Here's how the part is built. I have some questions about the finished solid (model axes, mm). Round coordinates to 2 decimals unless told otherwise and drop trailing zeros. Loops run counter-clockwise (first coordinate to the right, second up) from the corner with the lowest first, then second, coordinate; pieces in that order, holes last. Notation, with made-up numbers: M 70.25,-17.75 L 117.25,-17.75 A19 cw 117.25,5.25 Z; hole C 30,76.25 d4. An arc over 180 degrees is marked long. Use a Markdown table: item, result.
from build123d import *

# Parameters (mm, degrees)
F0_R     = 57.15
F0_R_2   = 20.32
F0_R_3   = 2.54
F1_DEPTH = 3.175


with BuildPart() as f1:
    # F0 (on Front) → F1 (new body)
    with BuildSketch(Plane.XZ):
        Circle(F0_R)
        with BuildLine():
            Line((-42.883825, -24.53093), (-42.543459, -17.032195))
            ThreePointArc((-42.543459, -17.032195), (-39.820724, -19.644048), (-36.333463, -21.084213))
            Line((-36.333463, -21.084213), (-42.883825, -24.53093))
        make_face(mode=Mode.SUBTRACT)
        with BuildLine():
            Line((-52.656993, -14.806859), (-48.735586, -8.406121))
            ThreePointArc((-48.735586, -8.406121), (-47.587931, -11.928695), (-45.255162, -14.806859))
            Line((-45.255162, -14.806859), (-52.656993, -14.806859))
        make_face(mode=Mode.SUBTRACT)
        with BuildLine():
            Line((-28.536372, -27.7573), (-32.257507, -21.238095))
            ThreePointArc((-32.257507, -21.238095), (-28.390723, -22.188544), (-24.455277, -21.582207))
            Line((-24.455277, -21.582207), (-28.536372, -27.7573))
        make_face(mode=Mode.SUBTRACT)
        with BuildLine():
            Line((-11.408226, -22.576399), (-18.505276, -20.131249))
            ThreePointArc((-18.505276, -20.131249), (-14.403329, -18.445306), (-11.408226, -15.174568))
            Line((-11.408226, -15.174568), (-11.408226, -22.576399))
        make_face(mode=Mode.SUBTRACT)
        with BuildLine():
            Line((-2.212769, -11.019517), (-9.630398, -12.170889))
            ThreePointArc((-9.630398, -12.170889), (-7.613739, -8.986542), (-6.894672, -5.286552))
            Line((-6.894672, -5.286552), (-2.212769, -11.019517))
        make_face(mode=Mode.SUBTRACT)
        with BuildLine():
            Line((-55.724405, 0), (-49.719241, 4.503874))
            ThreePointArc((-49.719241, 4.503874), (-50.727289, 0.088311), (-49.719241, -4.327252))
            Line((-49.719241, -4.327252), (-55.724405, 0))
        make_face(mode=Mode.SUBTRACT)
        with BuildLine():
            Line((-51.745173, 14.383817), (-44.247499, 14.746812))
            ThreePointArc((-44.247499, 14.746812), (-47.252569, 11.671197), (-48.718844, 7.628934))
            Line((-48.718844, 7.628934), (-51.745173, 14.383817))
        make_face(mode=Mode.SUBTRACT)
        with BuildLine():
            Line((-42.743142, 24.165609), (-36.361622, 20.213004))
            ThreePointArc((-36.361622, 20.213004), (-39.870209, 19.076412), (-42.743142, 16.763777))
            Line((-42.743142, 16.763777), (-42.743142, 24.165609))
        make_face(mode=Mode.SUBTRACT)
        with Locations((-28.347915, 0)):
            Circle(F0_R_2, mode=Mode.SUBTRACT)
        with BuildLine():
            Line((-2.37326, 7.45949), (-6.511062, 1.196466))
            ThreePointArc((-6.511062, 1.196466), (-6.73835, 6.076043), (-9.213608, 10.287341))
            Line((-9.213608, 10.287341), (-2.37326, 7.45949))
        make_face(mode=Mode.SUBTRACT)
        with BuildLine():
            Line((-12.167714, 22.883349), (-12.55219, 15.386746))
            ThreePointArc((-12.55219, 15.386746), (-15.311854, 18.527025), (-19.101316, 20.292545))
            Line((-19.101316, 20.292545), (-12.167714, 22.883349))
        make_face(mode=Mode.SUBTRACT)
        with BuildLine():
            Line((-28.363025, 27.663627), (-24.455277, 21.25454))
            ThreePointArc((-24.455277, 21.25454), (-28.363025, 21.998871), (-32.257507, 21.18799))
            Line((-32.257507, 21.18799), (-28.363025, 27.663627))
        make_face(mode=Mode.SUBTRACT)
        Circle(F0_R_3, mode=Mode.SUBTRACT)
    extrude(amount=F1_DEPTH)


solid = f1.part
1. Imagine slicing it at C-C, the plane x = 17. Write out the boundary of the cut face in (y, z) (3 decimals).
Answer sheet:
| item | result |
|---|---|
| outline | M -3.175,-54.563 L 0,-54.563 L 0,54.563 L -3.175,54.563 Z |
2. Imagine slicing it at D-D, the plane z = 34. Write out the boundary of the cut face in (x, y) (3 decimals), then the cut area to 3 significant figures.
Answer sheet:
| item | result |
|---|---|
| outline | M -45.936,-3.175 L 45.936,-3.175 L 45.936,0 L -45.936,0 Z |
| area | 292 mm2 |
3. Imagine slicing it at B-B, the plane y = -2.4. State how many separate pieces and enclosed holes the cut face has, then the cut area to 3 significant figures.
Answer sheet:
| item | result |
|---|---|
| separate pieces | 1 |
| enclosed holes | 13 |
| area | 8,720 mm2 |
4. We'd pull the mould along X, two halves only. Please class faces 1 (the face through (-57.095, -1.565, 2.513)), 2 (the face through (12, 0, 1)), 3 (the face through (-15.26, -1.57, 18.49)), 4 (the face through (-0.33, -1.57, 2.52)): +X half, -X half, draft (parallel to the pull), parting line (faces both ways), or undercut.
Answer sheet:
| item | result |
|---|---|
| face 1 | parting line |
| face 2 | draft |
| face 3 | undercut |
| face 4 | undercut |
5. I need wall thicknesses on probe 1 along Z at (x, y) = (0, -1.85); probe 2 along X at (y, z) = (-2.45, -14); probe 3 along X at (y, z) = (-3, 7). Which ranges of each line are inside material? Lowest first, please. Write a range as from..to.
Answer sheet:
| item | result |
|---|---|
| probe 1 | -57.15..-2.54, 2.54..57.15 |
| probe 2 | -55.41..-52.16, -46.1..-43.08, -13.62..55.41 |
| probe 3 | -56.72..-47.42, -9.27..-7.06, -2.68..56.72 |
6. For pin 1 Ø1.6 at (y, z) = (-2, 20.5) entering from +X; pin 2 Ø1 at (y, z) = (-1.5, -37) entering from -X; pin 3 Ø1 at (y, z) = (-0.5, 29) entering from -X, each with a flat end and sliding along its axis, tell me the tip position at first contact or that it passes through.
Answer sheet:
| item | result |
|---|---|
| pin 1 | x = 53.65 |
| pin 2 | x = -43.98 |
| pin 3 | x = -49.54 |
7. Imagine slicing it at A-A, the plane x = 0. Write out the boundary of the cut face in (y, z) (3 decimals).
Answer sheet:
| item | result |
|---|---|
| outline | M -3.175,-57.15 L 0,-57.15 L 0,-2.54 L -3.175,-2.54 Z; M -3.175,2.54 L 0,2.54 L 0,57.15 L -3.175,57.15 Z |
